from build123d import *

# Parameters (mm, degrees)
BOSS_EXTRUDE1_DEPTH = 25
FILLET3_R           = 5
FILLET4_R           = 5
FILLET6_R           = 5
FILLET7_R           = 5
SKETCH3_R           = 2
CUT_EXTRUDE1_DEPTH  = 10
SKETCH4_R           = 2.25
CUT_EXTRUDE2_DEPTH  = 10


with BuildPart() as part:
    # Sketch1 → Boss-Extrude1 (new body)
    with BuildSketch(Plane(origin=(0, 0, 0), x_dir=(1, 0, 0), z_dir=(0, 1, 0))):
        Polygon((-36.558892084, -26.613857404), (-36.558892084, -36.613857404), (48.441107916, -36.613857404), (43.778031334, -26.613857404), (48.203540535, -14.808578263), (46.184421194, -10.478562864), (44.37180562, -11.323799388), (45.545688437, -13.841199212), (39.201533928, -16.799527044), (-7.515811063, 83.386142596), (-16.578888933, 79.159959979), (0.325841536, 42.907648497), (6.669996046, 45.86597633), (23.574726515, 9.613664848), (17.230572006, 6.655337016), (26.404978218, -13.019240598), (21.456942355, -26.613857404), align=None)
    extrude(amount=BOSS_EXTRUDE1_DEPTH)

    # Fillet3
    fillet3_edges = [part.edges().sort_by_distance(p)[0] for p in [
        (-16.578888933, 12.5, -79.159959979),
    ]]
    fillet(fillet3_edges, radius=FILLET3_R)

    # Fillet4
    fillet4_edges = [part.edges().sort_by_distance(p)[0] for p in [
        (-36.558892084, 12.5, 26.613857404),
    ]]
    fillet(fillet4_edges, radius=FILLET4_R)

    # Fillet6
    fillet6_edges = [part.edges().sort_by_distance(p)[0] for p in [
        (23.574726515, 12.5, -9.613664848),
    ]]
    fillet(fillet6_edges, radius=FILLET6_R)

    # Fillet7
    fillet7_edges = [part.edges().sort_by_distance(p)[0] for p in [
        (6.669996046, 12.5, -45.86597633),
    ]]
    fillet(fillet7_edges, radius=FILLET7_R)

    # Sketch3 → Cut-Extrude1 (cut)
    with BuildSketch(Plane(origin=(25.765304939, 0, -12.014559008), x_dir=(-0.422618261740704, 0, -0.9063077870366479), z_dir=(0.9063077870366479, 0, -0.422618261740704))):
        with Locations((57.857173695, 12.5)):
            Circle(SKETCH3_R)
        with Locations((-7.792826305, 12.5)):
            Circle(SKETCH3_R)
    extrude(amount=-CUT_EXTRUDE1_DEPTH, mode=Mode.SUBTRACT)

    # Sketch4 → Cut-Extrude2 (cut)
    with BuildSketch(Plane.XY.offset(36.613857404)):
        with Locations((-21.558892084, 12.5)):
            Circle(SKETCH4_R)
        with Locations((13.441107916, 12.5)):
            Circle(SKETCH4_R)
    extrude(amount=-CUT_EXTRUDE2_DEPTH, mode=Mode.SUBTRACT)


solid = part.part
Can you work these out from the model? Positions are in its coordinate system, mm. A direction names the side the tool comes from. Round coordinates to 2 decimals unless told otherwise and drop trailing zeros. Loops run counter-clockwise (first coordinate to the right, second up) from the corner with the lowest first, then second, coordinate; pieces in that order, holes last. Notation, with made-up numbers: (58, 74) - (99, 74) arc R20 cw to (99, 90) - close; hole circle Ø6 at (25, 20). An arc over 180 degrees is marked (long way). Answer in a Markdown table with one row per item. Add a question column.
Q1. We'd pull the mould along Y, two halves only. Please class faces 4 (the flat face through (21.75, 12.32, 3.04)), 5 (the flat face through (18, 0, -6)), 6 (the cylindrical face through (-23.22, 14.02, 31.68)), 7 (the cylindrical face through (14.65, 14.4, 31.68)): pulls with the +Y half, pulls with the -Y half, needs draft (parallel to the pull), parting line crosses it, or undercut.
Q2. For pin 1 Ø5 at (x, y) = (-24.5, 11) entering from -Z; pin 2 Ø7 at (x, y) = (13.44, 12.5) entering from -Z; pin 3 Ø4 at (y, z) = (8.5, -17) entering from -X, each with a flat end and sliding along its axis, tell me the tip position at first contact or that it passes through.
Q3. I need wall thicknesses on L1, parallel to Z at x = -13.5, y = 16; L2, parallel to Z at x = 13.5, y = 2.5; L3, parallel to Y at x = -21, z = 28. Which ranges of each line are inside material? Lowest first, please.
Q4. I want a section at A-A on y = 7.25. List the corners of the cut face in (x, z) for me, and give its area (3 significant figures).
Q5. I want a section at B-B on x = 13. List the corners of the cut face in (y, z) for me, and give its area (3 significant figures).
Q6. Which directions (+Z, -Z, +X, -X, +Y, -Y) give clear straight access to the entire face, cutting with the end or side of a thin tool? Please do faces 1 (the flat face through (23.966, 12.325, 19.721)), 2 (the flat face through (42.42, 12.32, 15.3)), 3 (the flat face through (45.96, 12.32, 20.79)).
Q7. I want a section at D-D on y = 12.5. Count the separate pieces of the cut face and the enclosed holes in it, and give its area (3 significant figures).
Q8. I want a section at C-C on z = 29. List the corners of the cut face in (x, y) for me.
A:
| question | item | result |
|---|---|---|
| 1 | face 4 | needs draft |
| 1 | face 5 | pulls with the -Y half |
| 1 | face 6 | undercut |
| 1 | face 7 | undercut |
| 2 | pin 1 | z = 26.61 |
| 2 | pin 2 | z = -45.95 |
| 2 | pin 3 | x = 19.2 |
| 3 | L1 | -80.25 to -72.56, 26.61 to 36.61 |
| 3 | L2 | -38.32 to -31.22, 26.61 to 36.61 |
| 3 | L3 | 0 to 10.32, 14.68 to 25 |
| 4 | outline | (-36.56, 31.61) arc R5 ccw to (-31.56, 26.61) - (21.46, 26.61) - (26.4, 13.02) - (17.23, -6.66) - (19.04, -7.5) arc R5 cw to (21.46, -14.15) - (8.78, -41.33) arc R5 cw to (2.14, -43.75) - (0.33, -42.91) - (-14.47, -74.63) arc R5 ccw to (-12.05, -81.27) - (-7.52, -83.39) - (39.2, 16.8) - (45.55, 13.84) - (44.37, 11.32) - (46.18, 10.48) - (48.2, 14.81) - (43.78, 26.61) - (48.44, 36.61) - (-36.56, 36.61) - close |
| 4 | area | 1,880 mm^2 |
| 5 | outline | (0, -39.39) - (25, -39.39) - (25, -32.29) - (0, -32.29) - close; (0, 26.61) - (10.29, 26.61) - (10.29, 36.61) - (0, 36.61) - close; (14.71, 26.61) - (25, 26.61) - (25, 36.61) - (14.71, 36.61) - close |
| 5 | area | 383 mm^2 |
| 6 | face 1 | -X, +Y, -Y |
| 6 | face 2 | +Y, -Y |
| 6 | face 3 | +X, +Y, -Y |
| 7 | separate pieces | 5 |
| 7 | enclosed holes | 0 |
| 7 | area | 1,710 mm^2 |
| 8 | outline | (-35.82, 0) - (44.89, 0) - (44.89, 25) - (-35.82, 25) - close; hole circle Ø4.5 at (-21.56, 12.5); hole circle Ø4.5 at (13.44, 12.5) |
